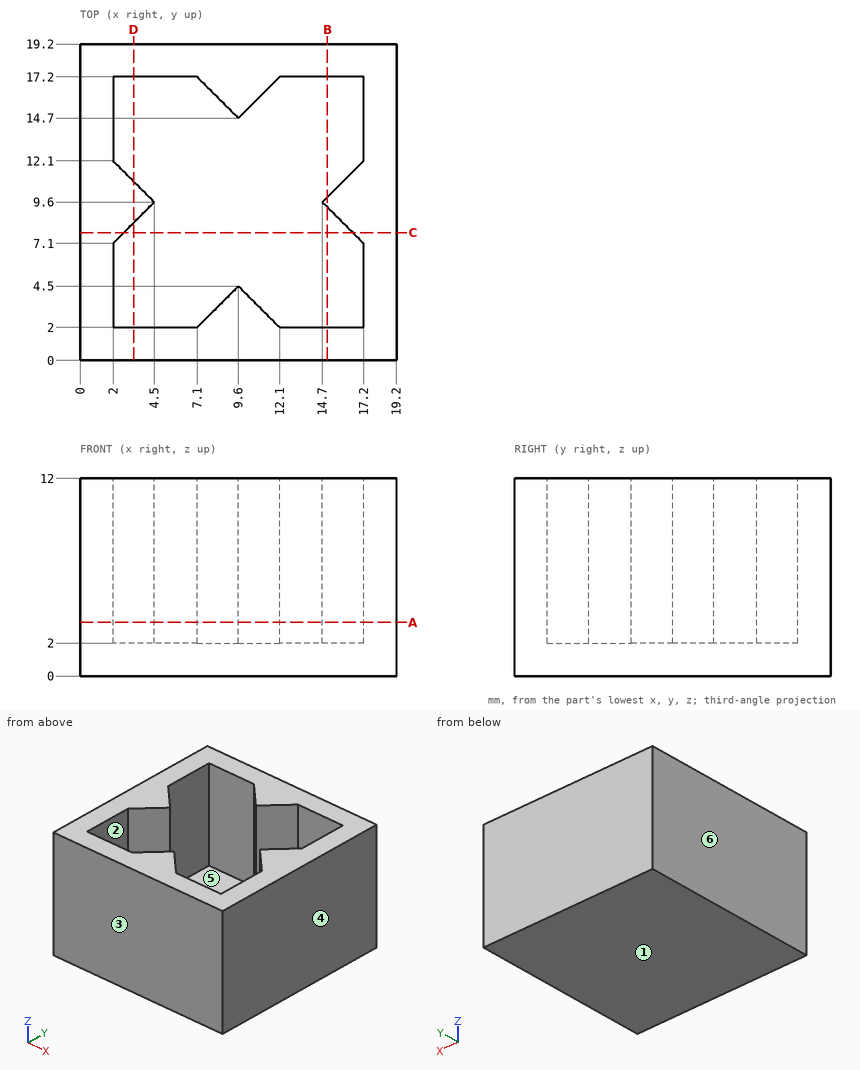
Study the drawing (mm; zero at the part's minimum x, y, z) and answer. A direction names the side the tool comes from. Coordinates: 2 decimals unless noted, no trailing zeros. Loops run counter-clockwise (first coordinate to the right, second up) from the corner with the lowest first, then second, coordinate; pieces in that order, holes last. Notation, with made-up numbers: (14, 72.25) -> (68, 72.25) arc R14 cw to (68, 80.25) -> close; hole circle Ø7 at (41.5, 26). An arc over 180 degrees is marked (long way). Answer as CSV lines item,"result".
1) The part is cut by section A-A (z = 3.25). Give the vertices of the cut face in (x, y), and give its area (3 significant figures).
A:
outline,"(0, 0) -> (19.2, 0) -> (19.2, 19.2) -> (0, 19.2) -> close; hole (2, 2) -> (7.1, 2) -> (9.6, 4.5) -> (12.1, 2) -> (17.2, 2) -> (17.2, 7.1) -> (14.7, 9.6) -> (17.2, 12.1) -> (17.2, 17.2) -> (12.1, 17.2) -> (9.6, 14.7) -> (7.1, 17.2) -> (2, 17.2) -> (2, 12.1) -> (4.5, 9.6) -> (2, 7.1) -> close"
area,"163 mm²"
2) The part is cut by section D-D (x = 3.25). Give the vertices of the cut face in (y, z), and give its area (3 significant figures).
A:
outline,"(0, 0) -> (19.2, 0) -> (19.2, 12) -> (17.2, 12) -> (17.2, 2) -> (10.85, 2) -> (10.85, 12) -> (8.35, 12) -> (8.35, 2) -> (2, 2) -> (2, 12) -> (0, 12) -> close"
area,"103 mm²"
3) For the marked faces 1 and 2, determine the directions among +Z, -Z, +X, -X, +Y, -Y from which every point of the face is accessible in a straight line to the end or side of a thin tool.
A:
face 1,"-Z, +X, -X, +Y, -Y"
face 2,"+Z"
4) Straight lines are drawn through the part: probe 1 along Y at (x, z) = (4.75, 2.25); probe 2 along Y at (x, z) = (17, 6.25). For each, find the intervals that lie inside material, in ascending order.
A:
probe 1,"y = 0 to 2, 17.2 to 19.2"
probe 2,"y = 0 to 2, 7.3 to 11.9, 17.2 to 19.2"
5) A flat-ended cylindrical pin translates along its axis: pin 1 (1.5 mm diameter, centred on x = 15.5, y = 3, fed in from +Z). Find the tip coordinate at first contact, or state that the pin passes through.
A:
pin 1,"stops at z = 2"
6) For a pull along X with two mould halves and no side action, classify the marked faces 3, 4, 5 and 6 as released by +X, released by -X, zero draft, split by the parting line, or undercut.
A:
face 3,"zero draft"
face 4,"released by +X"
face 5,"undercut"
face 6,"released by -X"
7) The part is cut by section B-B (x = 15). Give the vertices of the cut face in (y, z), and give its area (3 significant figures).
A:
outline,"(0, 0) -> (19.2, 0) -> (19.2, 12) -> (17.2, 12) -> (17.2, 2) -> (9.9, 2) -> (9.9, 12) -> (9.3, 12) -> (9.3, 2) -> (2, 2) -> (2, 12) -> (0, 12) -> close"
area,"84.4 mm²"
8) The part is cut by section C-C (y = 7.75). Give the vertices of the cut face in (x, z), and give its area (3 significant figures).
A:
outline,"(0, 0) -> (19.2, 0) -> (19.2, 12) -> (16.55, 12) -> (16.55, 2) -> (2.65, 2) -> (2.65, 12) -> (0, 12) -> close"
area,"91.4 mm²"
